For this review, take the finished solid that the model builds, in its own axes (mm). A direction names the side the tool comes from. Round coordinates to 2 decimals unless told otherwise and drop trailing zeros. Write each loop counter-clockwise with the first axis right and the second up, starting at its lowest first coordinate (ties: lowest second). Pieces come first, ordered by that corner, then holes. Notation, with made-up numbers: (-3.5, -33) -> (35.5, -33) arc R30 ccw to (35.5, -9) -> close; hole circle Ø9 at (36.25, 78.25). An arc over 180 degrees is marked (long way). Answer as CSV lines item,"result". Start each with the question number.
Item 1: Take a section at C-C on x = 37.5. Give the boundary of the cut face in (y, z), then the cut area to 3 significant figures.
Item 2: Take a section at B-B on z = 16. Give the boundary of the cut face in (x, y).
Item 3: Take a section at D-D on z = 45. Give the boundary of the cut face in (x, y).
Item 4: Machinability: for faces 1 (the cylindrical face through (57.385, 3.944, 6.751)), 2 (the flat face through (83, 18.5, 88)), 3 (the cylindrical face through (60.506, -2.465, 16.264)), 4 (the flat face through (75, 4, 44)), 5 (the cylindrical face through (64, 41, 87)), which of the approach directions +Z, -Z, +X, -X, +Y, -Y give a long, thin tool a straight path to every point of the face, cutting with its end or side? Answer none if there is none.
Item 5: Mouldability with a two-part tool opening along X and no side actions: class faces 6 (the cylindrical face through (2.85, 4.06, 86.99)), 7 (the cylindrical face through (124, 4, 79)), 8 (the flat face through (75, 30, 88)), 9 (the flat face through (108, 12, 88)) as +X half, -X half, draft (parallel to the pull), parting line (faces both ways), or undercut.
Item 6: For pin 1 Ø1.5 at (x, z) = (109.5, 88) entering from -Y; pin 2 Ø5 at (x, z) = (8.5, 74) entering from +Y; pin 3 Ø2.5 at (y, z) = (17, 88) entering from -X; pin 4 Ø6.5 at (x, z) = (8.5, 16) entering from -Y, all flat-tipped, find the tip position at first contact; note any pin that passes through.
Item 7: Take a section at A-A on x = 109.5. Give the boundary of the cut face in (y, z).
Item 8: Wall thickness on probe 1 along Z at (x, y) = (20, 5); probe 2 along Z at (x, y) = (66.5, -2.45); probe 3 along Z at (x, y) = (8, -3): over which ranges is each line inside the solid? List them lowest first. Write a range as from..to.
```python
from build123d import *

# Parameters (mm, degrees)
SKETCH1_W               = 75
SKETCH1_H               = 90
SKETCH1_W_2             = 50
SKETCH1_H_2             = 13
BOSS_EXTRUDE1_DEPTH     = 8
SKETCH2_R               = 18
SKETCH2_R_2             = 15.5
BOSS_EXTRUDE2_DEPTH     = 5
SKETCH3_R               = 2
CUT_EXTRUDE2_DEPTH      = 6
CUT_EXTRUDE2_DEPTH_BACK = 9
FILLET2_R               = 10
FILLET3_R               = 10
FILLET4_R               = 10
CUT_EXTRUDE3_REACH      = 10
SKETCH5_R               = 2.5
SKETCH7_W               = 5
SKETCH7_H               = 34
BOSS_EXTRUDE3_DEPTH     = 63
FILLET5_R               = 5
FILLET6_R               = 5
FILLET7_R               = 5
CUT_EXTRUDE4_REACH      = 92
SKETCH13_R              = 6
SKETCH13_R_2            = 2
BOSS_EXTRUDE4_DEPTH     = 5


with BuildPart() as part:
    # Sketch1 → Boss-Extrude1 (new body)
    with BuildSketch(Plane(origin=(0, 0, 0), x_dir=(1, 0, 0), z_dir=(0, 1, 0))):
        with Locations((37.5, -45)):
            Rectangle(SKETCH1_W, SKETCH1_H)
        with Locations((100, -83.5)):
            Rectangle(SKETCH1_W_2, SKETCH1_H_2)
    extrude(amount=BOSS_EXTRUDE1_DEPTH)

    # Sketch2 → Boss-Extrude2 (add)
    with BuildSketch(Plane.XZ):
        with Locations((37.5, 45)):
            Circle(SKETCH2_R)
        with Locations((37.5, 45)):
            Circle(SKETCH2_R_2, mode=Mode.SUBTRACT)
    extrude(amount=BOSS_EXTRUDE2_DEPTH)

    # Sketch3 → Cut-Extrude2 (cut, two sides)
    with BuildSketch(Plane.XZ) as cut_extrude2_sk:
        with Locations((8.5, 74)):
            Circle(SKETCH3_R)
        with Locations((66.5, 74)):
            Circle(SKETCH3_R)
        with Locations((8.5, 16)):
            Circle(SKETCH3_R)
        with Locations((66.5, 16)):
            Circle(SKETCH3_R)
    extrude(amount=CUT_EXTRUDE2_DEPTH, mode=Mode.SUBTRACT)
    extrude(cut_extrude2_sk.sketch, amount=-CUT_EXTRUDE2_DEPTH_BACK, mode=Mode.SUBTRACT)

    # Fillet2
    fillet2_edges = [part.edges().sort_by_distance(p)[0] for p in [
        (0, 4, 0),
    ]]
    fillet(fillet2_edges, radius=FILLET2_R)

    # Fillet3
    fillet3_edges = [part.edges().sort_by_distance(p)[0] for p in [
        (0, 4, 90),
    ]]
    fillet(fillet3_edges, radius=FILLET3_R)

    # Fillet4
    fillet4_edges = [part.edges().sort_by_distance(p)[0] for p in [
        (75, 4, 0),
    ]]
    fillet(fillet4_edges, radius=FILLET4_R)

    # Sketch5 → Cut-Extrude3 (cut, up to next)
    with BuildSketch(Plane.XZ, mode=Mode.PRIVATE) as cut_extrude3_sk1:
        with Locations((55, 6)):
            Circle(SKETCH5_R)
    cut_extrude3_tool1 = extrude(cut_extrude3_sk1.sketch, amount=-CUT_EXTRUDE3_REACH, mode=Mode.PRIVATE) & part.part
    add(cut_extrude3_tool1.solids().sort_by_distance((55, 0, 6))[0], mode=Mode.SUBTRACT)
    # Sketch5 → Cut-Extrude3 (cut, up to next)
    with BuildSketch(Plane.XZ, mode=Mode.PRIVATE) as cut_extrude3_sk2:
        with Locations((20, 84)):
            Circle(SKETCH5_R)
    cut_extrude3_tool2 = extrude(cut_extrude3_sk2.sketch, amount=-CUT_EXTRUDE3_REACH, mode=Mode.PRIVATE) & part.part
    add(cut_extrude3_tool2.solids().sort_by_distance((20, 0, 84))[0], mode=Mode.SUBTRACT)
    # Sketch5 → Cut-Extrude3 (cut, up to next)
    with BuildSketch(Plane.XZ, mode=Mode.PRIVATE) as cut_extrude3_sk3:
        with Locations((55, 84)):
            Circle(SKETCH5_R)
    cut_extrude3_tool3 = extrude(cut_extrude3_sk3.sketch, amount=-CUT_EXTRUDE3_REACH, mode=Mode.PRIVATE) & part.part
    add(cut_extrude3_tool3.solids().sort_by_distance((55, 0, 84))[0], mode=Mode.SUBTRACT)
    # Sketch5 → Cut-Extrude3 (cut, up to next)
    with BuildSketch(Plane.XZ, mode=Mode.PRIVATE) as cut_extrude3_sk4:
        with Locations((20, 6)):
            Circle(SKETCH5_R)
    cut_extrude3_tool4 = extrude(cut_extrude3_sk4.sketch, amount=-CUT_EXTRUDE3_REACH, mode=Mode.PRIVATE) & part.part
    add(cut_extrude3_tool4.solids().sort_by_distance((20, 0, 6))[0], mode=Mode.SUBTRACT)

    # Sketch7 → Boss-Extrude3 (add)
    with BuildSketch(Plane(origin=(125, 0, 0), x_dir=(0, 0, -1), z_dir=(1, 0, 0))):
        with Locations((-87.5, 25)):
            Rectangle(SKETCH7_W, SKETCH7_H)
    extrude(amount=-BOSS_EXTRUDE3_DEPTH)

    # Fillet5
    fillet5_edges = [part.edges().sort_by_distance(p)[0] for p in [
        (125, 42, 87.5),
    ]]
    fillet(fillet5_edges, radius=FILLET5_R)

    # Fillet6
    fillet6_edges = [part.edges().sort_by_distance(p)[0] for p in [
        (125, 4, 77),
    ]]
    fillet(fillet6_edges, radius=FILLET6_R)

    # Fillet7
    fillet7_edges = [part.edges().sort_by_distance(p)[0] for p in [
        (62, 42, 87.5),
    ]]
    fillet(fillet7_edges, radius=FILLET7_R)

    # Sketch12 → Cut-Extrude4 (cut, up to next)
    with BuildSketch(Plane.XY.offset(90), mode=Mode.PRIVATE) as cut_extrude4_sk1:
        with BuildLine():
            Line((77.5, 26.5), (87.5, 26.5))
            ThreePointArc((87.5, 26.5), (91.5, 22.5), (87.5, 18.5))
            Line((87.5, 18.5), (77.5, 18.5))
            ThreePointArc((77.5, 18.5), (73.5, 22.5), (77.5, 26.5))
        make_face()
    cut_extrude4_tool1 = extrude(cut_extrude4_sk1.sketch, amount=-CUT_EXTRUDE4_REACH, mode=Mode.PRIVATE) & part.part
    add(cut_extrude4_tool1.solids().sort_by_distance((82.5, 22.5, 90))[0], mode=Mode.SUBTRACT)
    # Sketch12 → Cut-Extrude4 (cut, up to next)
    with BuildSketch(Plane.XY.offset(90), mode=Mode.PRIVATE) as cut_extrude4_sk2:
        with BuildLine():
            Line((70.5, 33), (79.5, 33))
            ThreePointArc((79.5, 33), (81, 31.5), (79.5, 30))
            Line((79.5, 30), (70.5, 30))
            ThreePointArc((70.5, 30), (69, 31.5), (70.5, 33))
        make_face()
    cut_extrude4_tool2 = extrude(cut_extrude4_sk2.sketch, amount=-CUT_EXTRUDE4_REACH, mode=Mode.PRIVATE) & part.part
    add(cut_extrude4_tool2.solids().sort_by_distance((75, 31.5, 90))[0], mode=Mode.SUBTRACT)
    # Sketch12 → Cut-Extrude4 (cut, up to next)
    with BuildSketch(Plane.XY.offset(90), mode=Mode.PRIVATE) as cut_extrude4_sk3:
        with BuildLine():
            Line((70.5, 12), (79.5, 12))
            ThreePointArc((79.5, 12), (81, 13.5), (79.5, 15))
            Line((79.5, 15), (70.5, 15))
            ThreePointArc((70.5, 15), (69, 13.5), (70.5, 12))
        make_face()
    cut_extrude4_tool3 = extrude(cut_extrude4_sk3.sketch, amount=-CUT_EXTRUDE4_REACH, mode=Mode.PRIVATE) & part.part
    add(cut_extrude4_tool3.solids().sort_by_distance((75, 13.5, 90))[0], mode=Mode.SUBTRACT)
    # Sketch12 → Cut-Extrude4 (cut, up to next)
    with BuildSketch(Plane.XY.offset(90), mode=Mode.PRIVATE) as cut_extrude4_sk4:
        with BuildLine():
            Line((103.5, 33), (112.5, 33))
            ThreePointArc((112.5, 33), (114, 31.5), (112.5, 30))
            Line((112.5, 30), (103.5, 30))
            ThreePointArc((103.5, 30), (102, 31.5), (103.5, 33))
        make_face()
    cut_extrude4_tool4 = extrude(cut_extrude4_sk4.sketch, amount=-CUT_EXTRUDE4_REACH, mode=Mode.PRIVATE) & part.part
    add(cut_extrude4_tool4.solids().sort_by_distance((108, 31.5, 90))[0], mode=Mode.SUBTRACT)
    # Sketch12 → Cut-Extrude4 (cut, up to next)
    with BuildSketch(Plane.XY.offset(90), mode=Mode.PRIVATE) as cut_extrude4_sk5:
        with BuildLine():
            Line((103.5, 12), (112.5, 12))
            ThreePointArc((112.5, 12), (114, 13.5), (112.5, 15))
            Line((112.5, 15), (103.5, 15))
            ThreePointArc((103.5, 15), (102, 13.5), (103.5, 12))
        make_face()
    cut_extrude4_tool5 = extrude(cut_extrude4_sk5.sketch, amount=-CUT_EXTRUDE4_REACH, mode=Mode.PRIVATE) & part.part
    add(cut_extrude4_tool5.solids().sort_by_distance((108, 13.5, 90))[0], mode=Mode.SUBTRACT)

    # Sketch13 → Boss-Extrude4 (add)
    with BuildSketch(Plane.XZ):
        with Locations((8.5, 74)):
            Circle(SKETCH13_R)
        with Locations((8.5, 74)):
            Circle(SKETCH13_R_2, mode=Mode.SUBTRACT)
        with Locations((66.5, 74)):
            Circle(SKETCH13_R)
        with Locations((66.5, 74)):
            Circle(SKETCH13_R_2, mode=Mode.SUBTRACT)
        with Locations((66.5, 16)):
            Circle(SKETCH13_R)
        with Locations((66.5, 16)):
            Circle(SKETCH13_R_2, mode=Mode.SUBTRACT)
        with Locations((8.5, 16)):
            Circle(SKETCH13_R)
        with Locations((8.5, 16)):
            Circle(SKETCH13_R_2, mode=Mode.SUBTRACT)
    extrude(amount=BOSS_EXTRUDE4_DEPTH)


solid = part.part
```
Output values:
1,outline,"(-5, 27) -> (0, 27) -> (0, 0) -> (8, 0) -> (8, 90) -> (0, 90) -> (0, 63) -> (-5, 63) -> (-5, 60.5) -> (0, 60.5) -> (0, 29.5) -> (-5, 29.5) -> close"
1,area,"745 mm^2"
2,outline,"(0, 0) -> (2.5, 0) -> (2.5, -5) -> (6.5, -5) -> (6.5, 8) -> (0, 8) -> close; (10.5, -5) -> (14.5, -5) -> (14.5, 0) -> (60.5, 0) -> (60.5, -5) -> (64.5, -5) -> (64.5, 8) -> (10.5, 8) -> close; (68.5, -5) -> (72.5, -5) -> (72.5, 0) -> (75, 0) -> (75, 8) -> (68.5, 8) -> close"
3,outline,"(0, 0) -> (19.5, 0) -> (19.5, -5) -> (22, -5) -> (22, 0) -> (53, 0) -> (53, -5) -> (55.5, -5) -> (55.5, 0) -> (75, 0) -> (75, 8) -> (0, 8) -> close"
4,face 1,"+Y, -Y"
4,face 2,"+Z, -Z"
4,face 3,"-Y"
4,face 4,"-Z, +X, +Y, -Y"
4,face 5,"+Z, -Z, -X, +Y"
5,face 6,"-X half"
5,face 7,"+X half"
5,face 8,"undercut"
5,face 9,"undercut"
6,pin 1,"stops at y = 0"
6,pin 2,"stops at y = 8"
6,pin 3,"stops at x = 62"
6,pin 4,"stops at y = -5"
7,outline,"(0, 77) -> (8, 77) -> (8, 85) -> (12, 85) -> (12, 90) -> (0, 90) -> close; (15, 85) -> (30, 85) -> (30, 90) -> (15, 90) -> close; (33, 85) -> (42, 85) -> (42, 90) -> (33, 90) -> close"
8,probe 1,"z = 0..3.5, 8.5..81.5, 86.5..90"
8,probe 2,"z = 10..14, 18..22, 68..72, 76..80"
8,probe 3,"z = 10.02..14.06, 17.94..21.98, 68.02..72.06, 75.94..79.98"
